The figure shows three views and two pictorial views of one solid part (mm, origin at its lowest corner). Answer the questions. A direction names the side the tool comes from. Round coordinates to 2 decimals unless told otherwise and drop trailing zeros. Write each loop counter-clockwise with the first axis right and the second up, starting at its lowest first coordinate (ties: lowest second). Pieces come first, ordered by that corner, then holes. Notation, with made-up numbers: M 72,-2.75 L 81,-2.75 A15 ccw 81,10.25 Z; hole C -4.5,16.25 d1. An arc over 180 degrees is marked long. Answer in a Markdown table with one row per item.
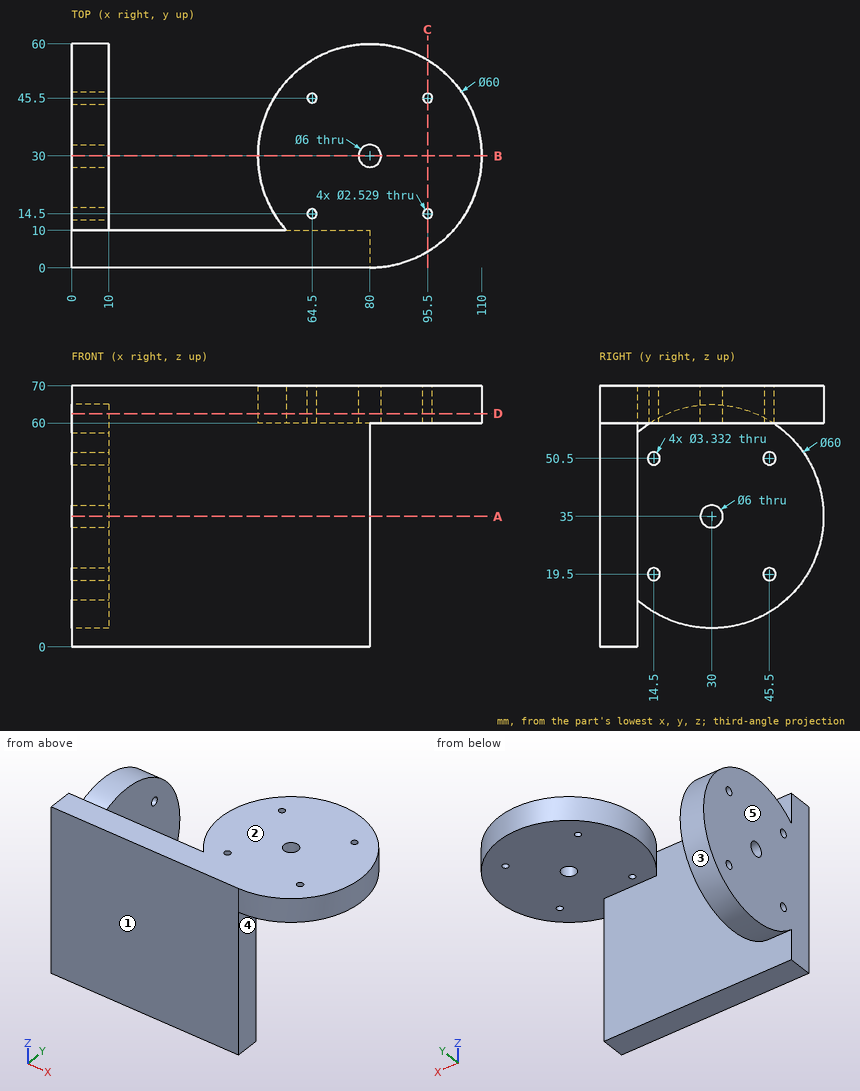
1. The part is cut by section D-D (z = 62.5). Determine the outline of the cut face in (x, y), plus the area to 3 significant figures.
Calculated:
| item | result |
|---|---|
| outline | M 0,0 L 80,0 A30 ccw long 57.64,10 L 0,10 Z; M 0,18.01 L 10,18.01 L 10,41.99 L 0,41.99 Z; hole C 64.5,14.5 d2.53; hole C 64.5,45.5 d2.53; hole C 80,30 d6; hole C 95.5,14.5 d2.53; hole C 95.5,45.5 d2.53 |
| area | 3,660 mm² |
2. Given pin 1 (4 mm diameter, centred on y = 30.5, z = 20.5, fed in from +X); pin 2 (3 mm diameter, centred on x = 44.5, z = 52, fed in from +Y); pin 3 (3.5 mm diameter, centred on x = 64.5, y = 45.5, fed in from -Z), each flat-ended and moving along its own axis, determine where each tip first touches the part or whether it passes through.
Calculated:
| item | result |
|---|---|
| pin 1 | stops at x = 10 |
| pin 2 | stops at y = 10 |
| pin 3 | stops at z = 60 |
3. The part is cut by section A-A (z = 35). Determine the outline of the cut face in (x, y).
Calculated:
| item | result |
|---|---|
| outline | M 0,0 L 80,0 L 80,10 L 10,10 L 10,27 L 0,27 Z; M 0,33 L 10,33 L 10,60 L 0,60 Z |
4. Determine the mould class of the marked faces 1, 2 and 3 for opening direction Y: released by +Y, released by -Y, zero draft, split by the parting line, or undercut.
Calculated:
| item | result |
|---|---|
| face 1 | released by -Y |
| face 2 | zero draft |
| face 3 | undercut |
5. Consider line 1 along Y through (x, z) = (64.5, 66.75); line 2 along X through (y, z) = (14.5, 67); line 3 along X through (y, z) = (27, 44). Determine where each line is inside the solid, lowest interval first. Write a range as from..to.
Calculated:
| item | result |
|---|---|
| line 1 | y = 0..13.24, 15.76..44.24, 46.76..55.69 |
| line 2 | x = 54.31..63.24, 65.76..94.24, 96.76..105.69 |
| line 3 | x = 0..10 |
6. The part is cut by section B-B (y = 30). Determine the outline of the cut face in (x, z), plus the area to 3 significant figures.
Calculated:
| item | result |
|---|---|
| outline | M 0,5 L 10,5 L 10,32 L 0,32 Z; M 0,38 L 10,38 L 10,65 L 0,65 Z; M 50,60 L 77,60 L 77,70 L 50,70 Z; M 83,60 L 110,60 L 110,70 L 83,70 Z |
| area | 1,080 mm² |
7. A tool of negligible diameter and unlimited length cuts with its end or side. For the marked faces 4 and 5, from which of +Z, -Z, +X, -X, +Y, -Y can it reach the whole face along a straight path? Write none if from no direction.
Calculated:
| item | result |
|---|---|
| face 4 | -Z, +X, +Y, -Y |
| face 5 | +Z, -Z, -X, +Y, -Y |
8. The part is cut by section C-C (x = 95.5). Determine the outline of the cut face in (y, z), plus the area to 3 significant figures.
Calculated:
| item | result |
|---|---|
| outline | M 4.31,60 L 13.24,60 L 13.24,70 L 4.31,70 Z; M 15.76,60 L 44.24,60 L 44.24,70 L 15.76,70 Z; M 46.76,60 L 55.69,60 L 55.69,70 L 46.76,70 Z |
| area | 463 mm² |
